Design review of the part built by this model. Coordinates are the model's own, in mm. A direction names the side the tool comes from. Give positions to 0.01 mm unless a question says otherwise; leave off trailing zeros. Order: outer loops, then holes, each group sorted by start corner. A loop starts at its lowest first (then second) coordinate and runs counter-clockwise, first axis right, second up. Notation, with made-up numbers: M -13.5,21 L 31.5,21 A10 cw 31.5,32 Z; hole C -18.5,60 d7. An arc over 180 degrees is marked long. Put each result on its own line as item: value. Start each with the question number.
from build123d import *

# Parameters (mm, degrees)
BOSS_EXTRUDE1_DEPTH = 12.7
FILLET1_R           = 1.27
FILLET2_R           = 0.635
SKETCH2_R           = 1.7
CUT_EXTRUDE1_DEPTH  = 22.120313829
SKETCH3_R           = 1.7
CUT_EXTRUDE2_DEPTH  = 22.120313829


with BuildPart() as part:
    # Sketch1 → Boss-Extrude1 (new body)
    with BuildSketch(Plane.XY):
        Polygon((0, 0), (0, 12.7), (1.5875, 12.7), (1.5875, 1.5875), (12.7, 1.5875), (12.7, 0), align=None)
    extrude(amount=BOSS_EXTRUDE1_DEPTH)

    # Fillet1
    fillet1_edges = [part.edges().sort_by_distance(p)[0] for p in [
        (1.5875, 1.5875, 6.35),
    ]]
    fillet(fillet1_edges, radius=FILLET1_R)

    # Fillet2
    fillet2_edges = [part.edges().sort_by_distance(p)[0] for p in [
        (1.5875, 12.7, 6.35),
        (12.7, 1.5875, 6.35),
    ]]
    fillet(fillet2_edges, radius=FILLET2_R)

    # Sketch2 → Cut-Extrude1 (cut, through all)
    with BuildSketch(Plane(origin=(1.5875, 0, 0), x_dir=(0, 0, -1), z_dir=(1, 0, 0))):
        with Locations(Location((-6.35, 7.46125, 0), (0, 0, 90))):
            Circle(SKETCH2_R)
    extrude(amount=-CUT_EXTRUDE1_DEPTH, mode=Mode.SUBTRACT)

    # Sketch3 → Cut-Extrude2 (cut, through all)
    with BuildSketch(Plane(origin=(0, 1.5875, 0), x_dir=(1, 0, 0), z_dir=(0, 1, 0))):
        with Locations(Location((7.46125, -6.35, 0), (0, 0, 270))):
            Circle(SKETCH3_R)
    extrude(amount=-CUT_EXTRUDE2_DEPTH, mode=Mode.SUBTRACT)


solid = part.part
1. Insertion check: pin 1 (2 mm diameter, centred on x = 7.46, z = 6.35, fed in from -Y); pin 2 (3 mm diameter, centred on y = 10, z = 6, fed in from +X); pin 3 (6 mm diameter, centred on x = 9, z = 10, fed in from +Y). Each pin has a flat end and moves straight along its axis. Give the tip position at first contact, or say it passes through.
2. To check wall thickness, follow probe 1 along X at (y, z) = (0.6, 6.35); probe 2 along X at (y, z) = (4.5, 4). State the ranges of each line that lie inside material, in increasing order.
3. Consider section C-C on x = 8.5. Give the boundary of the cut face in (y, z), then the cut area to 3 significant figures.
4. Consider section D-D on z = 3.5. Give the boundary of the cut face in (x, y) (1 decimal).
5. Machinability: for faces 4 (the cylindrical face through (9.147, 0.805, 6.129)), 5 (the flat face through (6, 1.588, 5)), which of the approach directions +Z, -Z, +X, -X, +Y, -Y give a long, thin tool a straight path to every point of the face, cutting with its end or side? Answer none if there is none.
6. Consider section B-B on y = 6.25. Give the boundary of the cut face in (x, z).
7. The part is to be moulded in two halves that separate along Z. For faces 1 (the flat face through (4, 1, 0)), 2 (the cylindrical face through (0.805, 7.24, 8.036)), 3 (the flat face through (0, 5, 6)), say which applies: +Z half, -Z half, draft (parallel to the pull), parting line (faces both ways), or undercut.
8. Consider section A-A on z = 6.35. Give the boundary of the cut face in (x, y) (1 decimal).
Returned:
1. pin 1: passes through
1. pin 2: stops at x = 1.59
1. pin 3: stops at y = 1.59
2. probe 1: x = 0 to 5.76, 9.16 to 12.7
2. probe 2: x = 0 to 1.59
3. outline: M 0,0 L 1.59,0 L 1.59,5 L 0,5 Z; M 0,7.7 L 1.59,7.7 L 1.59,12.7 L 0,12.7 Z
3. area: 15.9 mm2
4. outline: M 0,0 L 12.7,0 L 12.7,1 A0.6 ccw 12.1,1.6 L 2.9,1.6 A1.3 cw 1.6,2.9 L 1.6,12.1 A0.6 ccw 1,12.7 L 0,12.7 Z
5. face 4: +Y, -Y
5. face 5: +Z, -Z, +X, +Y
6. outline: M 0,0 L 1.59,0 L 1.59,5.16 L 0,5.16 Z; M 0,7.54 L 1.59,7.54 L 1.59,12.7 L 0,12.7 Z
7. face 1: -Z half
7. face 2: undercut
7. face 3: draft
8. outline: M 0,0 L 5.8,0 L 5.8,1.6 L 2.9,1.6 A1.3 cw 1.6,2.9 L 1.6,5.8 L 0,5.8 Z; M 0,9.2 L 1.6,9.2 L 1.6,12.1 A0.6 ccw 1,12.7 L 0,12.7 Z; M 9.2,0 L 12.7,0 L 12.7,1 A0.6 ccw 12.1,1.6 L 9.2,1.6 Z
